Input: dimensioned drawing with shaded views. Units: mm. Origin: part minimum x, y, z. A direction names the side the tool comes from. Coordinates: 2 decimals unless noted, no trailing zeros. Order: outer loops, then holes, each group sorted by start corner. A loop starts at its lowest first (then second) coordinate and runs counter-clockwise, first axis right, second up. Notation, with made-up numbers: M -21.5,65 L 24.5,65 A11 cw 24.5,81 Z; hole C 81,72.25 d10. An arc over 180 degrees is marked long. Use CSV: the item, a comma, the result in double quotes. Start each with the question number.
1. Section query C-C on y = 10. Return the cut outline in (x, z) (1 decimal).
2. Section query B-B on x = 45. Return the cut outline in (y, z).
3. First-contact query: P1, Ø15.5, axis at x = 20, y = 21, coming from the +Z side; P2, Ø6, axis at x = 20, z = 6, coming from the -Y side; P3, Ø4, axis at y = 11, z = 13, coming from the -X side (1 decimal); P4, Ø8.5, axis at y = 27.5, z = 8, coming from the -X side (1 decimal). Flat tips, straight axial feed; report the tip coordinate or a pass-through.
4. Pull-direction query (X, two-part tool) for the marked faces 3, 4 and 5; classes: pulls with the +X half, pulls with the -X half, needs draft (parallel to the pull), parting line crosses it, or undercut.
5. Set-up query: the marked faces 1 and 2. Return all of +Z, -Z, +X, -X, +Y, -Y with unobstructed straight access to the full face (end or side cutting, diameter ignored); none if empty.
6. Material intervals for line 1 (X direction, y = 16.5, z = 4.75); line 2 (X direction, y = 11, z = 7.75) (1 decimal); line 3 (X direction, y = 27.5, z = 11), sorted ascending.
7. Section query A-A on z = 5.5. State how many separate pieces and enclosed holes the cut face has, and give its area (3 significant figures).
8. Section query D-D on x = 25. Return the cut outline in (y, z).
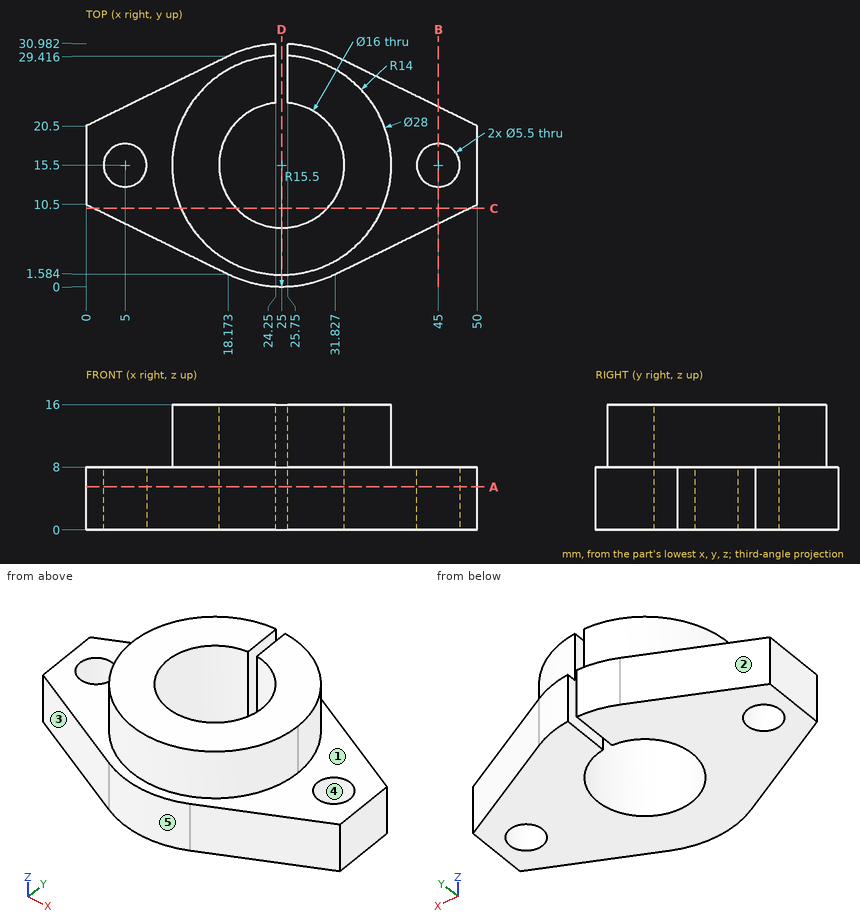
Results list:
1,outline,"M 1,0 L 19.2,0 L 19.2,16 L 12.1,16 L 12.1,8 L 1,8 Z; M 30.8,0 L 49,0 L 49,8 L 37.9,8 L 37.9,16 L 30.8,16 Z"
2,outline,"M 8.05,0 L 12.75,0 L 12.75,8 L 8.05,8 Z; M 18.25,0 L 22.95,0 L 22.95,8 L 18.25,8 Z"
3,P1,"stops at z = 16"
3,P2,"stops at y = 0.13"
3,P3,"stops at x = 11.2"
3,P4,"stops at x = 5.6"
4,face 3,"pulls with the -X half"
4,face 4,"undercut"
4,face 5,"parting line crosses it"
5,face 1,"+Z"
5,face 2,"+Z, -Z, -X, +Y"
6,line 1,"x = 0 to 2.44, 7.56 to 17.06, 32.94 to 42.44, 47.56 to 50"
6,line 2,"x = 0 to 18.4, 31.6 to 50"
6,line 3,"x = 17.79 to 24.25, 25.75 to 32.21"
7,separate pieces,"1"
7,enclosed holes,"2"
7,area,"837 mm²"
8,outline,"M 0,0 L 7.5,0 L 7.5,16 L 1.5,16 L 1.5,8 L 0,8 Z"
